Model file for the job. Use its own axes, mm. A direction names the side the tool comes from. Coordinates: 2 decimals unless noted, no trailing zeros. Order: outer loops, then holes, each group sorted by start corner. A loop starts at its lowest first (then second) coordinate and runs counter-clockwise, first axis right, second up. Notation, with made-up numbers: M 31,44 L 36,44 A13 cw 36,52 Z; hole C 40,-23.5 d1. An arc over 180 degrees is marked long. Return JSON: item names as keys, results as strings.
```python
from build123d import *

# Parameters (mm, degrees)
SKETCH_W      = 61.5
SKETCH_H      = 61.5
PAD_DEPTH     = 2
SKETCH001_W   = 61.5
SKETCH001_H   = 61.5
SKETCH001_W_2 = 57.9
SKETCH001_H_2 = 57.9
PAD001_DEPTH  = 19
SKETCH002_W   = 25
SKETCH002_H   = 25
PAD002_DEPTH  = 10
SKETCH003_R   = 2.3
POCKET_DEPTH  = 31.001


with BuildPart() as part:
    # Sketch → Pad (new body)
    with BuildSketch(Plane.XY):
        Rectangle(SKETCH_W, SKETCH_H)
    extrude(amount=PAD_DEPTH)

    # Sketch001 → Pad001 (new body)
    with BuildSketch(Plane(origin=(0, 0, 0), x_dir=(1, 0, 0), z_dir=(0, 0, -1))):
        Rectangle(SKETCH001_W, SKETCH001_H)
        Rectangle(SKETCH001_W_2, SKETCH001_H_2, mode=Mode.SUBTRACT)
    extrude(amount=PAD001_DEPTH)

    # Sketch002 → Pad002 (new body)
    with BuildSketch(Plane.XY.offset(2)):
        Rectangle(SKETCH002_W, SKETCH002_H)
    extrude(amount=PAD002_DEPTH)

    # Sketch003 → Pocket (cut, through all)
    with BuildSketch(Plane.XY.offset(12)):
        with Locations((-5.16188, 5.16188)):
            Circle(SKETCH003_R)
        with Locations((5.16188, -5.16188)):
            Circle(SKETCH003_R)
        with Locations((5.16188, 5.16188)):
            Circle(SKETCH003_R)
        with Locations((-5.16188, -5.16188)):
            Circle(SKETCH003_R)
    extrude(amount=-POCKET_DEPTH, mode=Mode.SUBTRACT)


solid = part.part
```
Item 1: Saw through at C-C (z = -5). Write the cut outline in (x, y).
Check result:
{"outline": "M -30.75,-30.75 L 30.75,-30.75 L 30.75,30.75 L -30.75,30.75 Z; hole M -28.95,-28.95 L 28.95,-28.95 L 28.95,28.95 L -28.95,28.95 Z"}
Item 2: Saw through at A-A (x = -11.5). Write the cut outline in (y, z), and give its area (3 significant figures).
Check result:
{"outline": "M -30.75,-19 L -28.95,-19 L -28.95,0 L 28.95,0 L 28.95,-19 L 30.75,-19 L 30.75,2 L 12.5,2 L 12.5,12 L -12.5,12 L -12.5,2 L -30.75,2 Z", "area": "441 mm2"}
Item 3: 3-axis set-ups, long thin cutter, end or side, ignore diameter. For faces 1 (the flat face through (-12.5, 0, 7)), 2 (the flat face through (0, -12.5, 7)), 3 (the flat face through (0, 12.5, 7)), 4 (the flat face through (28.95, 0, -9)): which of +Z, -Z, +X, -X, +Y, -Y reach the whole face in a straight line?
Check result:
{"face 1": "+Z, -X, +Y, -Y", "face 2": "+Z, +X, -X, -Y", "face 3": "+Z, +X, -X, +Y", "face 4": "-Z"}
Item 4: Pull direction X, two halves, no side cores. Call faces 5 (the flat face through (-28.95, 0, -9)), 6 (the flat face through (-30.75, 0, -8)), 7 (the flat face through (0, 30.75, -8)): +X half, -X half, draft (parallel to the pull), parting line (faces both ways), or undercut.
Check result:
{"face 5": "undercut", "face 6": "-X half", "face 7": "draft"}
Item 5: Drop flat-ended pins along their axis: pin 1 Ø3.5 at (x, y) = (5.16, -5.16) entering from -Z; pin 2 Ø5.5 at (x, y) = (5.16, 5.16) entering from -Z; pin 3 Ø5 at (y, z) = (5, 6.5) entering from +X; pin 4 Ø11 at (x, z) = (5.5, 6) entering from -Y. Give the stop position or say it passes through.
Check result:
{"pin 1": "passes through", "pin 2": "stops at z = 0", "pin 3": "stops at x = 12.5", "pin 4": "stops at y = -30.75"}
Item 6: Saw through at D-D (z = 4). Write the cut outline in (x, y).
Check result:
{"outline": "M -12.5,-12.5 L 12.5,-12.5 L 12.5,12.5 L -12.5,12.5 Z; hole C -5.16,-5.16 d4.6; hole C -5.16,5.16 d4.6; hole C 5.16,-5.16 d4.6; hole C 5.16,5.16 d4.6"}
Item 7: Wall check: line 1 (Y direction, x = 5, z = 7.5); line 2 (X direction, y = -12, z = -6.5); line 3 (X direction, y = 4.5, z = 7.5). Give the ranges that are in metal, low to high.
Check result:
{"line 1": "y = -12.5 to -7.46, -2.87 to 2.87, 7.46 to 12.5", "line 2": "x = -30.75 to -28.95, 28.95 to 30.75", "line 3": "x = -12.5 to -7.36, -2.96 to 2.96, 7.36 to 12.5"}
